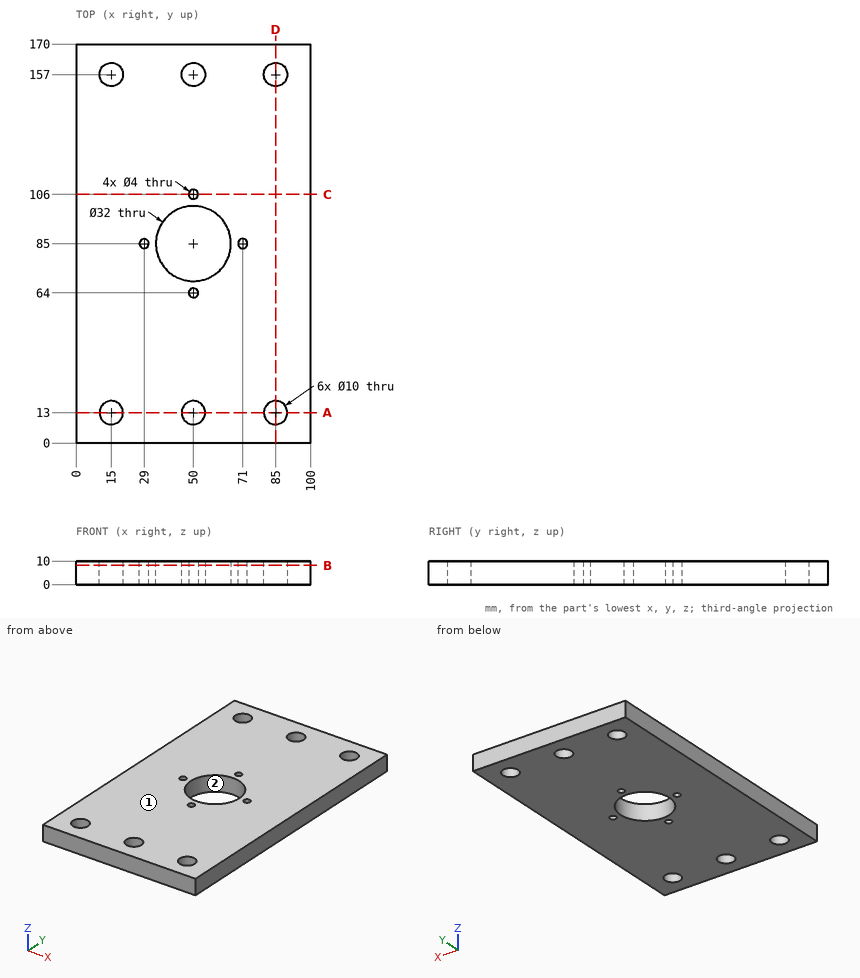
Geometry: see drawing. Coordinates: mm, zero at the bounding-box minimum. Coordinates: 2 decimals unless noted, no trailing zeros. Write each loop counter-clockwise with the first axis right and the second up, starting at its lowest first coordinate (ties: lowest second). Pieces come first, ordered by that corner, then holes.
1) Section A-A on y = 13. Output: boundary loops of the cut face in (x, z).
2) Pin query (flat end, axial travel): pin 1 Ø2.5 at (x, y) = (50, 64) entering from +Z; pin 2 Ø10 at (x, y) = (69, 149.5) entering from -Z. Return the tip coordinate at first contact, or that it passes through.
3) Mould query, pull axis X, two halves, no side actions, for the marked faces 1 and 2. Classes: pulls with the +X half, pulls with the -X half, needs draft (parallel to the pull), parting line crosses it, or undercut.
4) Section D-D on x = 85. Output: boundary loops of the cut face in (y, z).
5) Material intervals for line 1 along X through (y, z) = (157, 4.5); line 2 along Y through (x, z) = (85, 2.5); line 3 along Y through (x, z) = (17, 8.25), sorted ascending.
6) Section C-C on y = 106. Output: boundary loops of the cut face in (x, z).
7) Section B-B on z = 8.25. State how many separate pieces and enclosed holes the cut face has, and give its area (3 significant figures).
Check result:
1. outline: (0, 0) - (10, 0) - (10, 10) - (0, 10) - close; (20, 0) - (45, 0) - (45, 10) - (20, 10) - close; (55, 0) - (80, 0) - (80, 10) - (55, 10) - close; (90, 0) - (100, 0) - (100, 10) - (90, 10) - close
2. pin 1: passes through
2. pin 2: stops at z = 0
3. face 1: needs draft
3. face 2: undercut
4. outline: (0, 0) - (8, 0) - (8, 10) - (0, 10) - close; (18, 0) - (152, 0) - (152, 10) - (18, 10) - close; (162, 0) - (170, 0) - (170, 10) - (162, 10) - close
5. line 1: x = 0 to 10, 20 to 45, 55 to 80, 90 to 100
5. line 2: y = 0 to 8, 18 to 152, 162 to 170
5. line 3: y = 0 to 8.42, 17.58 to 152.42, 161.58 to 170
6. outline: (0, 0) - (48, 0) - (48, 10) - (0, 10) - close; (52, 0) - (100, 0) - (100, 10) - (52, 10) - close
7. separate pieces: 1
7. enclosed holes: 11
7. area: 15,700 mm2
